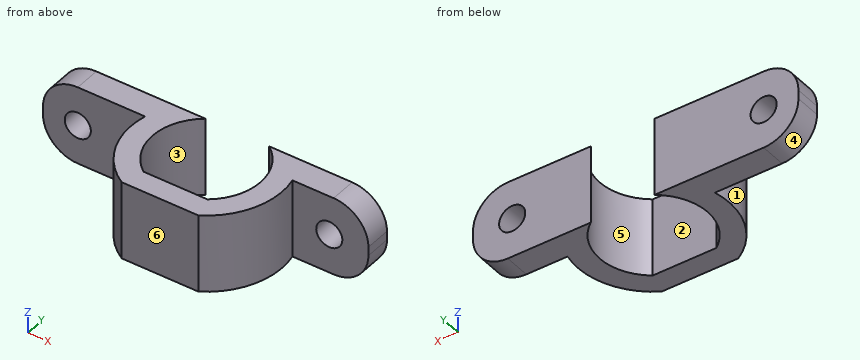
from build123d import *

# Parameters (mm, degrees)
BOSS_EXTRUDE1_DEPTH = 9
SKETCH2_R           = 1.5
CUT_EXTRUDE1_DEPTH  = 10
FILLET1_R           = 4


with BuildPart() as part:
    # Sketch1 → Boss-Extrude1 (new body)
    with BuildSketch(Plane.XY):
        with BuildLine():
            ThreePointArc((3.666060556, 5), (6.2, 0), (3.666060556, -5))
            Line((3.666060556, -5), (-3.666060556, -5))
            ThreePointArc((-3.666060556, -5), (-6.2, 0), (-3.666060556, 5))
            Line((-3.666060556, 5), (-20.2, 5))
            Line((-20.2, 5), (-20.2, 2))
            Line((-20.2, 2), (-8.466994744, 2))
            ThreePointArc((-8.466994744, 2), (-8.000677165, -3.41747932), (-4.409081537, -7.5))
            Line((-4.409081537, -7.5), (4.409081537, -7.5))
            ThreePointArc((4.409081537, -7.5), (8.000677165, -3.41747932), (8.466994744, 2))
            Line((8.466994744, 2), (17.2, 2))
            Line((17.2, 2), (17.2, 5))
            Line((17.2, 5), (3.666060556, 5))
        make_face()
    extrude(amount=BOSS_EXTRUDE1_DEPTH)

    # Sketch2 → Cut-Extrude1 (cut)
    with BuildSketch(Plane.XZ.offset(-2)):
        with Locations(Location((-16.2, 4.5, 0), (0, 0, 270))):
            Circle(SKETCH2_R)
        with Locations(Location((12.7, 4.5, 0), (0, 0, 270))):
            Circle(SKETCH2_R)
    extrude(amount=-CUT_EXTRUDE1_DEPTH, mode=Mode.SUBTRACT)

    # Fillet1
    fillet1_edges = [part.edges().sort_by_distance(p)[0] for p in [
        (-20.2, 3.5, 0),
        (17.2, 3.5, 0),
        (17.2, 3.5, 9),
        (-20.2, 3.5, 9),
    ]]
    fillet(fillet1_edges, radius=FILLET1_R)


solid = part.part
Could you check a few things on this model? Use its own coordinates, in mm. Face numbers are marked on the shaded views. A direction names the side the tool comes from. Give positions to 0.01 mm unless a question says otherwise; leave off trailing zeros. Order: outer loops, then holes, each group sorted by start corner. A loop starts at its lowest first (then second) coordinate and runs counter-clockwise, first axis right, second up.
1. Will these pins go through, and if not, where does the flat tip stop? P1, Ø1, axis at y = -2, z = 7.5, coming from the -X side; P2, Ø1.8, axis at x = -16.2, z = 4.5, coming from the +Y side; P3, Ø4, axis at x = 12.7, z = 4.5, coming from the -Y side; P4, Ø2, axis at x = -1.5, z = 5.5, coming from the +Y side.
2. Suppose I cut it at D-D (z = 1.5). List the corners of the cut face in (x, y) for me, plus the area to 3 significant figures.
3. Suppose I cut it at C-C (y = 1). List the corners of the cut face in (x, z) for me.
4. Suppose I cut it at B-B (x = 12.7). List the corners of the cut face in (y, z) for me.
5. Suppose I cut it at A-A (z = 4.5). List the corners of the cut face in (x, y) for me.
6. For the marked faces 1, 2 and 3, which set-ups out of +Z, -Z, +X, -X, +Y, -Y let a thin tool reach every point of the face, with its end or its side?
7. We'd pull the mould along X, two halves only. Please class the marked faces 4, 5 and 6: pulls with the +X half, pulls with the -X half, needs draft (parallel to the pull), parting line crosses it, or undercut.
8. I need wall thicknesses on L1, parallel to X at y = 3.1, z = 4.5; L2, parallel to X at y = 4.5, z = 3.75; L3, parallel to Y at x = -2.5, z = 4.5. Which ranges of each line are inside material? Lowest first, please.
Solved:
1. P1: stops at x = -8.57
1. P2: passes through
1. P3: stops at y = 2
1. P4: stops at y = -5
2. outline: (-19.32, 2) - (-8.47, 2) arc R8.7 ccw to (-4.41, -7.5) - (4.41, -7.5) arc R8.7 ccw to (8.47, 2) - (16.32, 2) - (16.32, 5) - (3.67, 5) arc R6.2 cw to (3.67, -5) - (-3.67, -5) arc R6.2 cw to (-3.67, 5) - (-19.32, 5) - close
2. area: 144 mm2
3. outline: (-8.64, 0) - (-6.12, 0) - (-6.12, 9) - (-8.64, 9) - close; (6.12, 0) - (8.64, 0) - (8.64, 9) - (6.12, 9) - close
4. outline: (2, 0) - (5, 0) - (5, 3) - (2, 3) - close; (2, 6) - (5, 6) - (5, 9) - (2, 9) - close
5. outline: (-20.2, 2) - (-17.7, 2) - (-17.7, 5) - (-20.2, 5) - close; (-14.7, 2) - (-8.47, 2) arc R8.7 ccw to (-4.41, -7.5) - (4.41, -7.5) arc R8.7 ccw to (8.47, 2) - (11.2, 2) - (11.2, 5) - (3.67, 5) arc R6.2 cw to (3.67, -5) - (-3.67, -5) arc R6.2 cw to (-3.67, 5) - (-14.7, 5) - close; (14.2, 2) - (17.2, 2) - (17.2, 5) - (14.2, 5) - close
6. face 1: +Z, -Z, -X
6. face 2: +Z, -Z, +Y
6. face 3: +Z, -Z
7. face 4: pulls with the -X half
7. face 5: undercut
7. face 6: needs draft
8. L1: x = -20.2 to -17.7, -14.7 to -5.37, 5.37 to 11.2, 14.2 to 17.2
8. L2: x = -20.19 to -17.5, -14.9 to -4.26, 4.26 to 11.4, 14 to 17.19
8. L3: y = -7.5 to -5
